Read the model definition and answer for the solid it produces. Units are mm, in the model's axes. Face numbers are marked on the shaded views. A direction names the side the tool comes from. Coordinates: 2 decimals unless noted, no trailing zeros. Loops run counter-clockwise (first coordinate to the right, second up) from the corner with the lowest first, then second, coordinate; pieces in that order, holes last. Notation, with made-up numbers: (46, 41.5) -> (101, 41.5) arc R24 ccw to (101, 80.5) -> close; hole circle Ø9 at (11.5, 20.5). An arc over 180 degrees is marked (long way). Answer as a JSON object with one key per item and string values. Group by question number.
Q1. The part is cut by section B-B on x = 161. Write down the section's boundary in (y, z), and give its area (3 significant figures).
Q2. The part is cut by section C-C on z = -75.5. Write down the section's boundary in (x, y), and give its area (3 significant figures).
Q3. The part is cut by section A-A on y = 151. Write down the section's boundary in (x, z), and give its area (4 significant figures).
Q4. Determine the mould class of the marked faces 1, 2, 3 and 4 for opening direction Y: released by +Y, released by -Y, zero draft, split by the parting line, or undercut.
Q5. For the marked faces 5 and 6, determine the directions among +Z, -Z, +X, -X, +Y, -Y from which every point of the face is accessible in a straight line to the end or side of a thin tool.
Q6. The part is cut by section D-D on x = 45.5. Write down the section's boundary in (y, z).
Q7. Straight lines are drawn through the part: line 1 along Y through (x, z) = (214.5, -41.5); line 2 along X through (y, z) = (52, -112.5); line 3 along Z through (x, y) = (110, 429). For each, find the intervals that lie inside material, in ascending order. Write a range as [from, to].
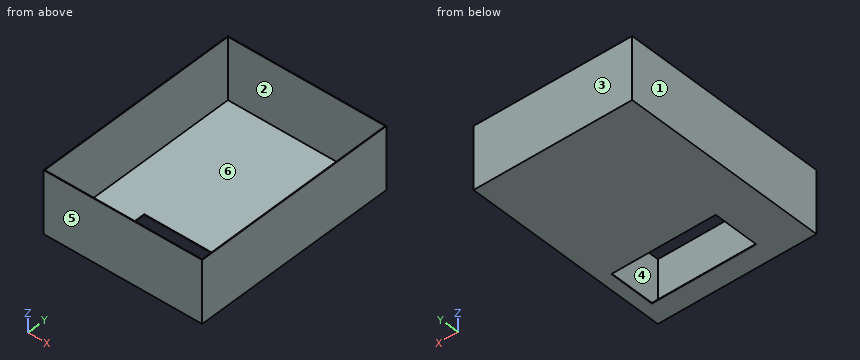
Autodesk Fusion 360 part; units mm, degrees
sketch "スケッチ1" plane through (0, 0, 0) normal (0, 1, 0) x (1, 0, 0)
  line L0 (0, 0) -> (380, 0)
  line L1 (380, 0) -> (380, 150)
  line L2 (380, 150) -> (0, 150)
  line L3 (0, 150) -> (0, 0)
  dimension "d1" = 380
  dimension "d2" = 150
extrude "押し出し1" add sketch "スケッチ1" along normal blind 500
sketch "スケッチ2" plane through (0, 0, 0) normal (0, 0, 1) x (1, 0, 0)
  line L0 (0, 0) -> (380, 0)
  line L1 (380, 0) -> (380, 500)
  line L2 (380, 500) -> (0, 500)
  line L3 (0, 500) -> (0, 0)
sketch "スケッチ3" plane through (0, 0, 0) normal (0, 0, 1) x (1, 0, 0)
  line L0 (380, 500) -> (0, 500)
  line L1 (380.7982, 500) -> (380.7982, 498.5)
  line L2 (0, 500) -> (0, 0)
  line L3 (0, 471) -> (1.5, 471)
  line L4 (1.5, 471) -> (1.5, 502)
  line L5 (380, 0) -> (380, 500)
  line L6 (380, 50) -> (378.5, 50)
  line L7 (378.5, 50) -> (377, 50)
  line L8 (0, 0) -> (380, 0)
  line L9 (361, 0) -> (361, 1.5)
  line L10 (378.5, 1.5) -> (1.5, 1.5)
  line L11 (1.5, 1.5) -> (1.5, 498.5115)
  line L12 (1.5, 498.5115) -> (378.5, 498.5115)
  line L13 (378.5, 498.5115) -> (378.5, 1.5)
  dimension "d5" = 1.5
  dimension "d6" = 1.5
  dimension "d7" = 1.5
  dimension "d10" = 1.5
extrude "押し出し2" cut sketch "スケッチ3" against normal blind 148.5 contours L4 L10 L11 L12 L13
sketch "スケッチ4" plane through (0, 0, -150) normal (0, 0, -1) x (-1, 0, 0)
  line L0 (-380, 0) -> (0, 0)
  line L1 (0, 0) -> (0, 500)
  line L2 (0, 500) -> (-380, 500)
  line L3 (-380, 500) -> (-380, 0)
  line L4 (0, 0) -> (-100, 0)
  line L5 (-100, 0) -> (-100, 50)
  line L6 (-100, 50) -> (-350, 50)
  line L7 (-350, 50) -> (-350, 160)
  line L8 (-350, 160) -> (-100, 160)
  line L9 (-100, 160) -> (-100, 50)
  dimension "d13" = 100
  dimension "d14" = 50
  dimension "d15" = 250
  dimension "d16" = 110
extrude "押し出し3" cut sketch "スケッチ4" against normal blind 30 contours L6 L7 L8 L9
sketch "スケッチ5" plane through (0, 0, 0) normal (0, 0, 1) x (1, 0, 0)
  curve L0
  curve L1
  curve L2
  curve L3
  curve A0
  dimension "d19" = 65
  dimension "d24" = 82
sketch "スケッチ6" plane through (0, 0, 0) normal (0, 0, 1) x (1, 0, 0)
sketch "スケッチ7" plane through (0, 0, 0) normal (0, 1, 0) x (1, 0, 0)
sketch "スケッチ8" plane through (0, 0, 0) normal (0, 0, 1) x (1, 0, 0)
  curve L0
  curve L1
  line L2 (378.5, 1.5) -> (1.5, 1.5)
  curve L3
  curve L4
  curve L5
  curve L6
  curve L7
  curve A0
  point P0 (83.5, 1.5)
  dimension "d26" = 20
  dimension "d27" = 20
  dimension "d28" = 30
  dimension "d29" = 30
  dimension "d30" = 50
sketch "スケッチ9" plane through (0, 0, 0) normal (0, 0, 1) x (1, 0, 0)
  curve L0
  curve L1
  curve L2
  curve L3
  point P0 (21.5, 1.5)
  point P1 (51.5, 1.5)
sketch "スケッチ10" plane through (0, 0, 0) normal (0, 0, 1) x (1, 0, 0)
  curve L0
  curve L1
  curve L2
  curve L3
  dimension "d31" = 100
  dimension "d32" = 80
Final values:
{
 "1": {"outline": "(0, -150) -> (50, -150) -> (50, -148.5) -> (1.5, -148.5) -> (1.5, 0) -> (0, 0) -> close; (160, -150) -> (500, -150) -> (500, 0) -> (498.51, 0) -> (498.51, -148.5) -> (160, -148.5) -> close", "area": "1,030 mm2"},
 "2": {"outline": "(0, 0) -> (380, 0) -> (380, 500) -> (0, 500) -> close; hole (1.5, 1.5) -> (378.5, 1.5) -> (378.5, 498.51) -> (1.5, 498.51) -> close", "area": "2,630 mm2"},
 "3": {"outline": "(0, -150) -> (100, -150) -> (100, -148.5) -> (1.5, -148.5) -> (1.5, 0) -> (0, 0) -> close; (350, -150) -> (380, -150) -> (380, 0) -> (378.5, 0) -> (378.5, -148.5) -> (350, -148.5) -> close", "area": "640.5 mm2"},
 "4": {"face 1": "zero draft", "face 2": "undercut", "face 3": "released by +Y", "face 4": "undercut"},
 "5": {"face 5": "+Z, -Z, +X, -X, -Y", "face 6": "+Z"},
 "6": {"outline": "(0, -150) -> (500, -150) -> (500, 0) -> (498.51, 0) -> (498.51, -148.5) -> (1.5, -148.5) -> (1.5, 0) -> (0, 0) -> close"},
 "7": {"line 1": "y = [0, 1.5], [498.51, 500]", "line 2": "x = [0, 1.5], [378.5, 380]", "line 3": "z = [-150, -148.5]"}
}
